CAD build for the part. Positions are in the model's coordinates, mm. A direction names the side the tool comes from. Round coordinates to 2 decimals unless told otherwise and drop trailing zeros. Loops run counter-clockwise (first coordinate to the right, second up) from the corner with the lowest first, then second, coordinate; pieces in that order, holes last. Notation, with made-up numbers: (-8, 33) -> (41, 33) arc R20 cw to (41, 71) -> close; hole circle Ø4 at (19.5, -9). An arc over 180 degrees is marked (long way). Answer as CSV lines item,"result".
```python
from build123d import *

# Parameters (mm, degrees)
F0_W     = 101.6
F0_H     = 50.8
F1_DEPTH = 25.4
F2_R     = 6.35
F3_DEPTH = 25.401
F4_W     = 12.7
F4_H     = 25.4
F6_W     = 10.16
F6_H     = 6.35
F8_R     = 2.53999
F9_SIZE  = 2.54


# Not quite as in the source:
# - a fillet or chamfer is up to 0.001 mm smaller than in the source, because OpenCascade refuses the exact size


with BuildPart() as f1:
    # F0 (on Front) → F1 (new body)
    with BuildSketch(Plane.XZ):
        Rectangle(F0_W, F0_H)
    extrude(amount=F1_DEPTH)

    # F2 (on face) → F3 (cut, through all)
    with BuildSketch(Plane.XZ.offset(25.4)):
        with Locations((-38.1, 12.7)):
            Circle(F2_R)
        with Locations((-38.1, -12.7)):
            Circle(F2_R)
        with Locations((38.1, 12.7)):
            Circle(F2_R)
        with Locations((38.1, -12.7)):
            Circle(F2_R)
    extrude(amount=-F3_DEPTH, mode=Mode.SUBTRACT)

    # F4 (on Top) → F5 (revolve)
    with BuildSketch(Plane.XY):
        with Locations((-6.35, -38.1)):
            Rectangle(F4_W, F4_H)
    revolve(axis=Axis((0, -38.1, 0), (0, -1, 0)))

    # F6 (on Top) → F7 (revolve, cut)
    with BuildSketch(Plane.XY):
        with Locations((-15.24, -38.735)):
            Rectangle(F6_W, F6_H)
    revolve(axis=Axis((0, -57.4092715979, 0), (0, -1, 0)), mode=Mode.SUBTRACT)

    # F8 (radius 2.54 in the source; OpenCascade refuses exactly that, so slightly less here)
    f8_edges = [f1.edges().sort_by_distance(p)[0] for p in [
        (12.7, -25.4, 0),
        (10.16, -35.56, 0),
        (10.16, -41.91, 0),
        (-10.16, -38.735, 0),
    ]]
    fillet(f8_edges, radius=F8_R)

    # F9
    f9_edges = [f1.edges().sort_by_distance(p)[0] for p in [
        (-50.8, -25.4, 0),
        (0, -25.4, 25.4),
        (50.8, -25.4, 0),
        (0, -25.4, -25.4),
    ]]
    chamfer(f9_edges, length=F9_SIZE)


solid = f1.part
```
Q1. Two-plate mould, pull along Z, no slides. Class faces 1 (the flat face through (49.55, -24.11, -0.36)), 2 (the cylindrical face through (2.75, -46.29, 12.4)), 3 (the cylindrical face through (-32.234, -12.878, -15.132)): pulls with the +Z half, pulls with the -Z half, needs draft (parallel to the pull), parting line crosses it, or undercut.
Results:
face 1,"needs draft"
face 2,"parting line crosses it"
face 3,"undercut"
Q2. Drop flat-ended pins along their axis: pin 1 Ø7.5 at (x, z) = (38.1, -12.7) entering from +Y; pin 2 Ø3 at (x, z) = (26, 5.5) entering from -Y; pin 3 Ø1.5 at (y, z) = (-30, -3) entering from +X. Give the stop position or say it passes through.
Results:
pin 1,"through"
pin 2,"y = -25.4"
pin 3,"x = 12.5"
Q3. Slice it at D-D, the plane z = 17. Give the cut face in (x, y), and give its area (3 significant figures).
Results:
outline,"(-50.8, -22.86) -> (-48.26, -25.4) -> (-42.77, -25.4) -> (-42.77, 0) -> (-50.8, 0) -> close; (-33.43, -25.4) -> (33.43, -25.4) -> (33.43, 0) -> (-33.43, 0) -> close; (42.77, -25.4) -> (48.26, -25.4) -> (50.8, -22.86) -> (50.8, 0) -> (42.77, 0) -> close"
area,"2,100 mm2"
Q4. Probe L1, parallel to Z at x = 38.1, y = -19.5; L2, parallel to X at y = -6.5, z = 12.5; L3, parallel to X at y = -9, z = 18.5. List the from-to ranges inside material, lowest first. Write a range as [from, to].
Results:
L1,"[-25.4, -19.05], [-6.35, 6.35], [19.05, 25.4]"
L2,"[-50.8, -44.45], [-31.75, 31.75], [44.45, 50.8]"
L3,"[-50.8, -40.69], [-35.51, 35.51], [40.69, 50.8]"
Q5. Slice it at B-B, the plane y = -21.5. Give the cut face in (x, z).
Results:
outline,"(-50.8, -25.4) -> (50.8, -25.4) -> (50.8, 25.4) -> (-50.8, 25.4) -> close; hole circle Ø12.7 at (-38.1, -12.7); hole circle Ø12.7 at (-38.1, 12.7); hole circle Ø12.7 at (38.1, -12.7); hole circle Ø12.7 at (38.1, 12.7)"
Q6. Tool access for faces 4 (the flat face through (-1, -11, -25.4)), 5 (the cylindrical face through (2.75, -31.7, 12.4)), 6 (the cylindrical face through (1.323, -38.726, -10.074)): list every direction of +Z, -Z, +X, -X, +Y, -Y with a clear straight run to the whole face (end or side of a thin tool).
Results:
face 4,"-Z, +X, -X, +Y, -Y"
face 5,"-Y"
face 6,"none"
Q7. Slice it at A-A, the plane x = 38.1. Give the cut face in (y, z), and give its area (3 significant figures).
Results:
outline,"(-25.4, -22.86) -> (-22.86, -25.4) -> (0, -25.4) -> (0, -19.05) -> (-25.4, -19.05) -> close; (-25.4, -6.35) -> (0, -6.35) -> (0, 6.35) -> (-25.4, 6.35) -> close; (-25.4, 19.05) -> (0, 19.05) -> (0, 25.4) -> (-22.86, 25.4) -> (-25.4, 22.86) -> close"
area,"639 mm2"
